Geometry check sheet. Reference: the model listing, model coordinates, mm. Face numbers are marked on the shaded views. A direction names the side the tool comes from. Round coordinates to 2 decimals unless told otherwise and drop trailing zeros. Order: outer loops, then holes, each group sorted by start corner. A loop starts at its lowest first (then second) coordinate and runs counter-clockwise, first axis right, second up. Notation, with made-up numbers: (7, 45) -> (44, 45) arc R26 ccw to (44, 73) -> close; hole circle Ø4 at (71.25, 30.25). An arc over 180 degrees is marked (long way). Use a Markdown table: item, result. Add a question column.
Item 1: Set-up check for the marked faces 1 and 2: record each of +Z, -Z, +X, -X, +Y, -Y from which the full face is reachable in a straight line by a thin tool's end or side.
Item 2: Sectioned sample at A-A, the plane y = 0. Record the cut outline in (x, z).
Item 3: Sectioned sample at C-C, the plane z = 10.5. Record the cut outline in (x, y).
Item 4: Sectioned sample at B-B, the plane x = 5. Record the cut outline in (y, z).
Item 5: Sectioned sample at D-D, the plane x = 0.25. Record the cut outline in (y, z).
Item 6: Material ranges on probe 1 along Z at (x, y) = (1.25, -0.5); probe 2 along X at (y, z) = (-0.05, 5.75); probe 3 along X at (y, z) = (0.35, 3.25), recorded low to high. Write a range as [from, to].
from build123d import *

# Parameters (mm, degrees)
SKETCH1_R           = 0.79375
BOSS_EXTRUDE1_DEPTH = 19.304
BOSS_EXTRUDE5_START = -1.27
BOSS_EXTRUDE5_DEPTH = 1.27


with BuildPart() as part:
    # Sketch1 → Boss-Extrude1 (new body)
    with BuildSketch(Plane.XY):
        Circle(SKETCH1_R)
    extrude(amount=BOSS_EXTRUDE1_DEPTH)

    # Sketch3 → Boss-Extrude5 (add)
    with BuildSketch(Plane.XY.offset(19.304).offset(BOSS_EXTRUDE5_START)):
        with BuildLine():
            Line((0, 0.79375), (6.35, 0.79375))
            ThreePointArc((6.35, 0.79375), (7.14375, 0), (6.35, -0.79375))
            Line((6.35, -0.79375), (0, -0.79375))
            ThreePointArc((0, -0.79375), (-0.79375, 0), (0, 0.79375))
        make_face()
    extrude(amount=BOSS_EXTRUDE5_DEPTH)


solid = part.part
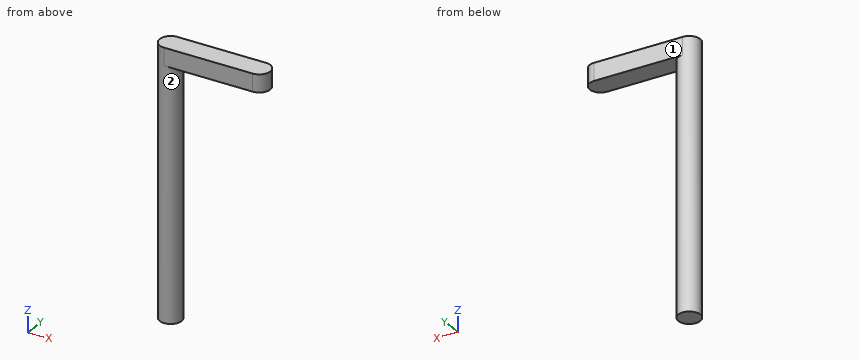
Found:
| question | item | result |
|---|---|---|
| 1 | face 1 | +Z, -Z, +X, -X, +Y |
| 1 | face 2 | -Z |
| 2 | outline | (-0.79, 0) -> (0.79, 0) -> (0.79, 18.03) -> (7.14, 18.03) -> (7.14, 19.3) -> (-0.79, 19.3) -> close |
| 3 | outline | circle Ø1.59 at (0, 0) |
| 4 | outline | (-0.79, 18.03) -> (0.79, 18.03) -> (0.79, 19.3) -> (-0.79, 19.3) -> close |
| 5 | outline | (-0.79, 18.03) -> (-0.75, 18.03) -> (-0.75, 0) -> (0.75, 0) -> (0.75, 18.03) -> (0.79, 18.03) -> (0.79, 19.3) -> (-0.79, 19.3) -> close |
| 6 | probe 1 | z = [18.03, 19.3] |
| 6 | probe 2 | x = [-0.79, 0.79] |
| 6 | probe 3 | x = [-0.71, 0.71] |
